Geometry check sheet. Reference: the model listing, model coordinates, mm. A direction names the side the tool comes from. Give positions to 0.01 mm unless a question says otherwise; leave off trailing zeros. Loops run counter-clockwise (first coordinate to the right, second up) from the corner with the lowest first, then second, coordinate; pieces in that order, holes last. Notation, with made-up numbers: (50.5, 74) -> (64.5, 74) arc R5 ccw to (64.5, 78) -> close; hole circle Ø4 at (-4.75, -36). An arc over 180 degrees is marked (long way). Write each question's results on one line, items separated by ' | '. Start each with the question number.
1) Scan lines: line 1 (Y direction, x = -19, z = 0.75) (3 decimals); line 2 (Y direction, x = 0, z = 4.25) (3 decimals); line 3 (Z direction, x = -7.5, y = -2.25). Record each from-to range of solid material in increasing order. Write a range as from..to.
2) Sectioned sample at C-C on y = -2. Record the cut outline in (x, z) (3 decimals), then the cut area to 3 significant figures.
3) Depth check by flat-ended pin: pin 1 (3 mm diameter, centred on x = -12, y = -3, fed in from -Z); pin 2 (1 mm diameter, centred on y = -4, z = 2, fed in from +X); pin 3 (5.5 mm diameter, centred on x = -12, y = 0, fed in from +Z); pin 4 (1.5 mm diameter, centred on y = -7, z = 2.5, fed in from +X). Enter the tip coordinate at first touch or a pass-through.
4) Set-up check for faces 5 (the face through (-3.532, -5.435, 4.74)), 6 (the face through (-5.287, 2.76, 5.143)), 7 (the face through (-14.58, -0.18, 1.57)): record each of +Z, -Z, +X, -X, +Y, -Y from which the full face is reachable in a straight line by a thin tool's end or side.
5) Draft check along Y on faces 1 (the face through (-3, -9, 3.175)), 2 (the face through (0.06, -7.61, 1.57)), 3 (the face through (-7.32, -3.23, 5.14)), 4 (the face through (-0.31, 1.39, 3.13)). Enter one of: pulls with the +Y half, pulls with the -Y half, needs draft (parallel to the pull), parting line crosses it, or undercut.
6) Sectioned sample at D-D on x = -11.5. Record the cut outline in (y, z) (3 decimals).
7) Sectioned sample at A-A on y = 0.75. Record the cut outline in (x, z).
Autodesk Inventor part; units mm, degrees
ref_plane "YZ Plane" through (0, 0, 0) normal (1, 0, 0) x (0, 1, 0)
ref_plane "XZ Plane" through (0, 0, 0) normal (0, 1, 0) x (-1, 0, 0)
ref_plane "XY Plane" through (0, 0, 0) normal (0, 0, 1) x (1, 0, 0)
sketch "Sketch1" plane through (0, 0, 0) normal (0, 0, 1) x (1, 0, 0)
  circle A0 centre (0, 0) radius 1.4224
  circle A1 centre (0, 0) radius 3.175
  line L0 (0, 0) -> (-19.05, 0) construction
  circle A2 centre (-2.476506, -10.833032) radius 3.175
  circle A3 centre (-2.476506, -10.833032) radius 5 construction
  circle A4 centre (-2.476506, -10.833032) radius 1.5
  line L1 (0, 0) -> (-2.476506, -10.833032) construction
  line L2 (-2.476506, -10.833032) -> (-3.938782, -10.498745) construction
  line L3 (0, 0) -> (-2.476506, -10.833032) construction
  arc A5 (-5.54332, -10.011281) -> (0.590309, -11.654782) centre (-2.476506, -10.833032) ccw
  arc A6 (-1.02973, -3.003378) -> (-19.05, 0) centre (-19.05, -55.5625) ccw
  arc A7 (-19.05, 3.175) -> (-19.05, 0) centre (-19.05, 1.5875) ccw
  line L4 (-19.05, 3.175) -> (0, 3.175)
  line L5 (-2.476506, -10.833032) -> (-4.878131, 0) construction
  line L6 (0.623234, -10.145836) -> (-1.778391, 0.687196)
  line L7 (-7.977871, -0.687196) -> (-5.576246, -11.520227)
  arc A8 (-5.576246, -11.520227) -> (0.623234, -10.145836) centre (-2.476506, -10.833032) ccw
  arc A9 (-1.778391, 0.687196) -> (-7.977871, -0.687196) centre (-4.878131, 0) ccw
  circle A10 centre (6.746875, -0.79375) radius 3.175
  circle A11 centre (6.746875, -0.79375) radius 1.5
  line L8 (7.117846, 2.359503) -> (0.370971, 3.153253)
  arc A12 (4.720646, -3.238136) -> (-0.236744, -6.266728) centre (2.761054, -5.602132) ccw
  circle A13 centre (6.746875, -0.79375) radius 5 construction
  point P0 (0.590309, -11.654782)
  point P1 (0, 3.175)
  point P2 (-7.878677, -1.134631)
  point P3 (-5.576246, -11.520227)
  point P4 (0.623234, -10.145836)
  point P5 (-0.954741, -3.028051)
  point P6 (-2.439066, 2.03263)
  point P7 (1.235308, -2.924832)
  point P8 (1.403608, -2.847896)
  point P9 (-1.424341, -1.064207)
  point P10 (-1.702423, 0.512874)
  point P11 (0.623234, -10.145836)
  point P12 (-5.576246, -11.520227)
  dimension "d24" = 3
  dimension "d0" = 2.8448
  dimension "d1" = 6.35
  dimension "d9" = 19.05
  dimension "d22" = 6.35
  dimension "d23" = 10
  dimension "d26" = 11.1125
  dimension "d29" = 3.175
  dimension "d30" = 6.35
  dimension "d31" = 6.35
  dimension "d32" = 3
  dimension "d36" = 10
  dimension "d37" = 102.5
  dimension "d38" = 4.7625
  dimension "d39" = 6.74688
  dimension "d40" = 0.79375
sketch "Sketch1 outline for Extrusion1" plane through (0, 0, 0) normal (0, 0, 1) x (1, 0, 0)
  arc A0 (-19.05, 3.175) -> (-19.05, 0) centre (-19.05, 1.5875) ccw
  arc A1 (-19.05, 0) -> (-7.878677, -1.134631) centre (-19.05, -55.5625) cw
  line L0 (-7.878677, -1.134631) -> (-5.576246, -11.520227)
  arc A2 (-5.576246, -11.520227) -> (0.623234, -10.145836) centre (-2.476506, -10.833032) ccw
  line L1 (0.623234, -10.145836) -> (-0.954741, -3.028051)
  arc A3 (-0.954741, -3.028051) -> (0, 3.175) centre (0, 0) ccw
  line L2 (0, 3.175) -> (-19.05, 3.175)
  circle A4 centre (0, 0) radius 1.4224
  circle A5 centre (-2.476506, -10.833032) radius 1.5
extrude "Extrusion1" add sketch "Sketch1 outline for Extrusion1" along normal blind 3.175
fillet "Fillet1" radius 3.175 1 edges at (-7.8787, -1.1346, 1.5875)
sketch "Sketch2" plane through (0, 0, 3.175) normal (0, 0, 1) x (1, 0, 0)
  circle A0 centre (-2.476506, -10.833032) radius 1.5
  arc A1 (-0.348803, -5.761259) -> (-6.548283, -7.13565) centre (-2.476506, -10.833032) ccw
  line L0 (0, 3.175) -> (-19.05, 3.175)
  arc A2 (-19.05, 3.175) -> (-19.05, 0) centre (-19.05, 1.5875) ccw
  arc A3 (-10.006813, -0.74086) -> (-19.05, 0) centre (-19.05, -55.5625) ccw
  arc A4 (-7.423826, -3.18633) -> (-10.006813, -0.74086) centre (-10.523566, -3.873526) ccw
  line L1 (-7.423826, -3.18633) -> (-5.576246, -11.520227)
  arc A5 (-5.576246, -11.520227) -> (0.623234, -10.145836) centre (-2.476506, -10.833032) ccw
  line L2 (0.623234, -10.145836) -> (-0.954741, -3.028051)
  arc A6 (-0.954741, -3.028051) -> (0, 3.175) centre (0, 0) ccw
  circle A7 centre (0, 0) radius 1.4224
  circle A8 centre (-2.476506, -10.833032) radius 1.5
  arc A9 (-7.423826, -3.18633) -> (-10.006813, -0.74086) centre (-10.523566, -3.873526) ccw
  line L3 (0, 3.175) -> (-19.05, 3.175)
  arc A10 (-7.423826, -3.18633) -> (-5.7158, 3.175) centre (-18.4158, 3.175) ccw
  line L4 (0.623234, -10.145836) -> (-0.954741, -3.028051)
  line L5 (-7.423826, -3.18633) -> (-5.576246, -11.520227)
  point P0 (-6.548283, -7.13565)
  point P1 (-5.7158, 3.175)
  point P2 (-0.348803, -5.761259)
  dimension "d41" = 11
  dimension "d42" = 12.7
extrude "Extrusion2" add sketch "Sketch2" along normal blind 0.79375 contours A1 L1 A10 L0 A6 L2 | A4 A3 A2 L0 A10
extrude "Extrusion3" add sketch "Sketch2" along normal blind 3.175 contours A1 L1 A10 L0 A6 L2
fillet "Fillet2" radius 1.5875 5 edges at (-6.5483, -7.1357, 4.7625) (-7.4238, -3.1863, 5.1594) (-5.7158, 3.175, 5.1594) (-0.9547, -3.0281, 3.175) (-0.3488, -5.7613, 4.7625)
properties part number "Lever" material "Aluminum 6061"
Result:
1) line 1: 0..3.175 | line 2: -3.442..-1.422, 1.422..3.175 | line 3: 0..3.97
2) outline: (-7.96, 0) -> (2.466, 0) -> (2.466, 6.35) -> (-6.818, 6.35) -> (-6.818, 3.969) -> (-7.96, 3.969) -> close | area: 63.5 mm^2
3) pin 1: through | pin 2: x = -0.06 | pin 3: z = 3.97 | pin 4: x = 0.09
4) face 5: +Z, -Y | face 6: +Z, -X, +Y | face 7: +Z, -Z, -X, -Y
5) face 1: needs draft | face 2: undercut | face 3: parting line crosses it | face 4: undercut
6) outline: (-0.515, 0) -> (3.175, 0) -> (3.175, 3.969) -> (-0.515, 3.969) -> close
7) outline: (-20.4, 0) -> (-1.21, 0) -> (-1.21, 6.35) -> (-5.95, 6.35) -> (-5.95, 3.97) -> (-20.4, 3.97) -> close; (1.21, 0) -> (3.09, 0) -> (3.09, 6.35) -> (1.21, 6.35) -> close
